from build123d import *

# Parameters (mm, degrees)
BOSS_EXTRUDE1_DEPTH     = 95.25
CUT_EXTRUDE1_DEPTH      = 120.305668348
CUT_EXTRUDE1_DEPTH_BACK = 120.305668348


with BuildPart() as part:
    # Sketch1 → Boss-Extrude1 (new body)
    with BuildSketch(Plane(origin=(0, 0, 0), x_dir=(1, 0, 0), z_dir=(0, 1, 0))):
        Polygon((50.8, 0), (0, 0), (0, -50.8), (12.7, -50.8), (26.645567884, -26.645567884), (50.8, -12.7), align=None)
    extrude(amount=BOSS_EXTRUDE1_DEPTH)

    # Sketch2 → Cut-Extrude1 (cut, two sides: drawn at the far end of the back side and taken through both)
    with BuildSketch(Plane.XY.offset(-CUT_EXTRUDE1_DEPTH_BACK)):
        Polygon((-151.156603976, 263.126416075), (0, 95.25), (50.8, 38.830884247), (201.956603976, -129.045531829), (537.709436127, 173.267676124), (184.596228174, 565.439624028), align=None)
    extrude(amount=CUT_EXTRUDE1_DEPTH + CUT_EXTRUDE1_DEPTH_BACK, mode=Mode.SUBTRACT)


solid = part.part
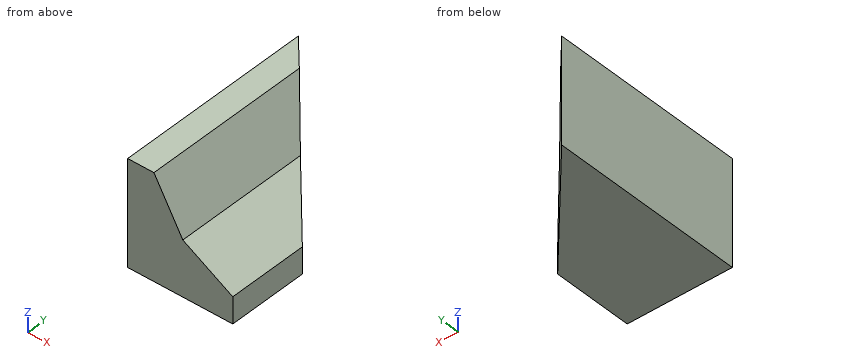
Geometry check sheet. Reference: the model listing, model coordinates, mm. Give positions to 0.01 mm unless a question says otherwise; leave off trailing zeros. Loops run counter-clockwise (first coordinate to the right, second up) from the corner with the lowest first, then second, coordinate; pieces in that order, holes last.
(1) Section check B-B on z = 10.5. Record the cut outline in (x, y).
From the geometry:
outline: (0, 0) - (50.8, 0) - (50.8, 38.83) - (0, 95.25) - close
(2) Section check D-D on y = 69.5. Record the cut outline in (x, z), then the cut area to 3 significant figures.
From the geometry:
outline: (0, 0) - (23.19, 0) - (23.19, 32.64) - (12.7, 50.8) - (0, 50.8) - close
area: 1,080 mm2
(3) Depth check by flat-ended pin: pin 1 Ø5 at (y, z) = (81.5, 26) entering from +X; pin 2 Ø8 at (x, y) = (37.5, 46.5) entering from +Z; pin 3 Ø3 at (y, z) = (48.5, 34) entering from +X. Enter the tip coordinate at first touch or a pass-through.
From the geometry:
pin 1: stops at x = 14.63
pin 2: stops at z = 22.69
pin 3: stops at x = 23.27
(4) Thickness scan on L1, parallel to X at y = 41.5, z = 41.5; L2, parallel to X at y = 78.5, z = 43; L3, parallel to Y at x = 38, z = 6. Record the ranges inside material, lowest first.
From the geometry:
L1: x = 0 to 18.07
L2: x = 0 to 15.08
L3: y = 0 to 53.05
(5) Section check A-A on y = 13.5. Record the cut outline in (x, z), then the cut area to 3 significant figures.
From the geometry:
outline: (0, 0) - (50.8, 0) - (50.8, 12.7) - (26.65, 26.65) - (12.7, 50.8) - (0, 50.8) - close
area: 1,660 mm2
(6) Section check C-C on x = 8.5. Record the cut outline in (y, z).
From the geometry:
outline: (0, 0) - (85.81, 0) - (85.81, 50.8) - (0, 50.8) - close
